Autodesk Inventor part; units mm, degrees
ref_plane "Work Plane1" through (3, 0, 0) normal (0, 0, 1) x (1, 0, 0)
ref_plane "YZ Plane" through (0, 0, 0) normal (1, 0, 0) x (0, 1, 0)
ref_plane "XZ Plane" through (0, 0, 0) normal (0, 1, 0) x (-1, 0, 0)
sketch "Sketch1" plane through (0, 0, 0) normal (0, 0, 1) x (1, 0, 0)
  line L0 (0, 0) -> (2.8333, 0)
  line L1 (6, 1.1547) -> (6, 2)
  line L2 (6, 2) -> (0, 2)
  line L3 (6, 1.1547) -> (3.5, 1.1547)
  line L4 (3.5, 1.1547) -> (2.8333, 0)
  line L5 (0, -0.4) -> (0, 2.4)
  line L6 (0, 2) -> (0, 0)
  dimension "d0" = 2.5
  dimension "d1" = 60
  dimension "d2" = 4
  dimension "d3" = 2.3094
  dimension "d5" = 6
revolve "Body" add sketch "Sketch1" angle 360 about axis through (0, 0, 0) along (1, 0, 0)
sketch "Sketch2" plane through (6, 0, 0) normal (1, 0, 0) x (0, 1, 0)
  circle A0 centre (0, 0) radius 1.1547
  line L0 (-0.5774, 1) -> (0.5774, 1)
  line L1 (0.5774, 1) -> (1.1547, 0)
  line L2 (1.1547, 0) -> (0.5774, -1)
  line L3 (0.5774, -1) -> (-0.5774, -1)
  line L4 (-0.5774, -1) -> (-1.1547, 0)
  line L5 (-1.1547, 0) -> (-0.5774, 1)
  point P0 (0, 0)
  point P1 (0, 0)
extrude "Slot" add sketch "Sketch2" against normal up to next contours L1 A0 | A0 L2 | L0 A0 | A0 L3 | L5 A0 | A0 L4
thread "Thread"
chamfer "Chamfer1" distance 1.5 angle 45 1 edges at (0, -2, 0) measured on face at (4, 1.9741, -0.3208)
chamfer "Chamfer2" distance 0.4294 angle 45 1 edges at (6, -2, 0) measured on face at (4.5, 1.9741, -0.3208)
ref_plane "Work Plane1" through (3, 0, 0) normal (0, 0, 1) x (1, 0, 0)
equation "\"d0\" = INTI"
equation "\"d2\" = NND"
equation "\"d3\" = 1.1547 * SW"
equation "\"d5\" = NLG"
equation "\"d12\" = NLG"
equation "\"d9\" = FAWI"
equation "\"d10\" = -0.5 * GD1 + 0.5 * NND"
equation "\"d11\" = FAWI"
equation "\"d35\" = -0.5 * GD1 + 0.5 * NND"
equation "\"NND\" = 4"
equation "\"NLG\" = 6"
equation "\"INTI\" = 2.5"
equation "\"FAWI\" = 45deg"
equation "\"SW\" = 2"
equation "\"GD1\" = THREADDIA - 1.2269 * PTC"
equation "\"FAWI1\" = 45deg"
equation "\"SPD\" = 1"
equation "\"GUL\" = 0.61345 * PTC"
equation "\"TOA\" = 30deg"
equation "\"THREADDIA\" = 4"
equation "\"PTC\" = 0.7"
equation "\"GAL\" = 0.61345 * PTC"
equation "\"E0\" = 1.155 * SW"
properties part number "ISO 4027 - M4 x 6" material "Stainless Steel, 440C"
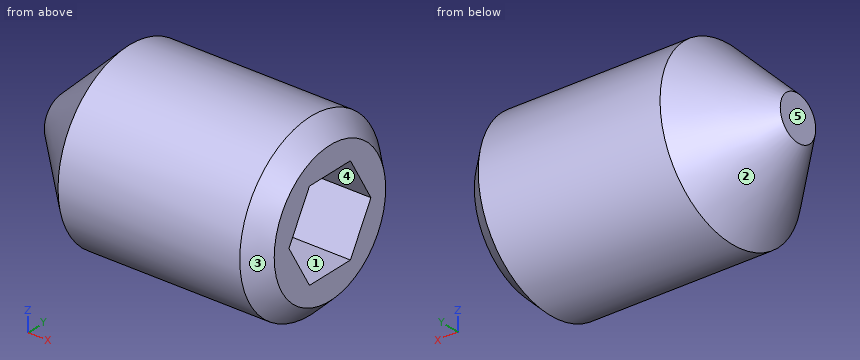
Could you check a few things on this model? Use its own coordinates, in mm. Face numbers are marked on the shaded views. A direction names the side the tool comes from. Coordinates: 2 decimals unless noted, no trailing zeros. Loops run counter-clockwise (first coordinate to the right, second up) from the corner with the lowest first, then second, coordinate; pieces in that order, holes last. Notation, with made-up numbers: (82, -25.75) -> (94, -25.75) arc R21 ccw to (94, 4.25) -> close; hole circle Ø3 at (12, -6.5). An arc over 180 degrees is marked (long way). Answer in a Markdown table with one row per item.
(1) Imagine slicing it at D-D (x = 2.95). List the corners of the cut face in (y, z) for me, plus the area to 3 significant figures.
Results found:
| item | result |
|---|---|
| outline | circle Ø4 at (0, 0); hole circle Ø0.4 at (0, 0) |
| area | 12.4 mm^2 |
(2) Imagine slicing it at B-B (x = 2.2). List the corners of the cut face in (y, z) for me.
Results found:
| item | result |
|---|---|
| outline | circle Ø4 at (0, 0) |
(3) Imagine slicing it at A-A (x = 4.7). List the corners of the cut face in (y, z) for me.
Results found:
| item | result |
|---|---|
| outline | circle Ø4 at (0, 0); hole (-1.15, 0) -> (-0.58, -1) -> (0.58, -1) -> (1.15, 0) -> (0.58, 1) -> (-0.58, 1) -> close |
(4) Thinking about a two-plate mould opening in Y: for the marked faces 3, 4 and 5, which applies, released by +Y, released by -Y, zero draft, split by the parting line, or undercut?
Results found:
| item | result |
|---|---|
| face 3 | split by the parting line |
| face 4 | undercut |
| face 5 | zero draft |
(5) For the marked faces 1 and 2, which set-ups out of +Z, -Z, +X, -X, +Y, -Y let a thin tool reach every point of the face, with its end or its side?
Results found:
| item | result |
|---|---|
| face 1 | +X |
| face 2 | -X |
(6) If I drill on probe 1 along Z at (x, y) = (5.55, 0.8); probe 2 along Y at (x, z) = (5.4, -0.6); probe 3 along Z at (x, y) = (4.4, -1.1), over which ranges is the centre line in solid material (lowest first)?
Results found:
| item | result |
|---|---|
| probe 1 | z = -1.83 to -0.61, 0.61 to 1.83 |
| probe 2 | y = -1.91 to -0.81, 0.81 to 1.91 |
| probe 3 | z = -1.67 to -0.09, 0.09 to 1.67 |
(7) Will these pins go through, and if not, where does the flat tip stop? pin 1 Ø1 at (x, z) = (5, -1.5) entering from -Y; pin 2 Ø2 at (x, z) = (2.5, -0.5) entering from +Y.
Results found:
| item | result |
|---|---|
| pin 1 | stops at y = -1.73 |
| pin 2 | stops at y = 2 |
(8) Imagine slicing it at C-C (x = 0.5). List the corners of the cut face in (y, z) for me.
Results found:
| item | result |
|---|---|
| outline | circle Ø2 at (0, 0) |
